Check sheet for the modelled part. Datum: model origin and axes. Units: mm. A direction names the side the tool comes from. Give positions to 0.01 mm unless a question says otherwise; leave off trailing zeros. Order: outer loops, then holes, each group sorted by start corner. A loop starts at its lowest first (then second) coordinate and runs counter-clockwise, first axis right, second up. Notation, with made-up numbers: M -33,18 L 4,18 A11 ccw 4,29 Z; hole C 58,48 d8. An arc over 180 degrees is marked long. Return JSON: item names as keys, results as strings. Group by question number.
from build123d import *

# Parameters (mm, degrees)
SKETCH1_W           = 6.35
SKETCH1_H           = 19.05
BOSS_EXTRUDE1_DEPTH = 1.5875
SKETCH2_W           = 5.2832
SKETCH2_H           = 4.7625
CUT_EXTRUDE1_DEPTH  = 1.5875
SKETCH3_R           = 0.762
SKETCH3_R_2         = 1.2573
CUT_EXTRUDE2_DEPTH  = 3.175
SKETCH31_R          = 2.54
CUT_EXTRUDE5_DEPTH  = 1.778


with BuildPart() as part:
    # Sketch1 → Boss-Extrude1 (new body, symmetric)
    with BuildSketch(Plane(origin=(0, 0, 0), x_dir=(1, 0, 0), z_dir=(0, 1, 0))):
        Polygon((-3.175, 15.08125), (-14.44625, 15.08125), (-14.44625, -15.08125), (-9.16305, -15.08125), (-9.16305, 5.55625), (9.16305, 5.55625), (9.16305, -15.08125), (14.44625, -15.08125), (14.44625, 15.08125), (3.175, 15.08125), align=None)
        with Locations((0, 24.60625)):
            Rectangle(SKETCH1_W, SKETCH1_H)
    extrude(amount=BOSS_EXTRUDE1_DEPTH, both=True)

    # Sketch2 → Cut-Extrude1 (cut)
    with BuildSketch(Plane(origin=(0, 1.5875, 0), x_dir=(1, 0, 0), z_dir=(0, 1, 0))):
        with Locations((-11.80465, -12.7)):
            Rectangle(SKETCH2_W, SKETCH2_H)
        with Locations((11.80465, -12.7)):
            Rectangle(SKETCH2_W, SKETCH2_H)
    extrude(amount=-CUT_EXTRUDE1_DEPTH, mode=Mode.SUBTRACT)

    # Sketch3 → Cut-Extrude2 (cut)
    with BuildSketch(Plane(origin=(0, 1.5875, 0), x_dir=(1, 0, 0), z_dir=(0, 1, 0))):
        with Locations((-11.65225, -12.7)):
            Circle(SKETCH3_R)
        with Locations((11.65225, -12.7)):
            Circle(SKETCH3_R)
        with Locations((0, 17.294029814)):
            Circle(SKETCH3_R_2)
        with Locations((0, 29.994029814)):
            Circle(SKETCH3_R_2)
    extrude(amount=-CUT_EXTRUDE2_DEPTH, mode=Mode.SUBTRACT)

    # Sketch31 → Cut-Extrude5 (cut)
    with BuildSketch(Plane(origin=(0, 1.5875, 0), x_dir=(1, 0, 0), z_dir=(0, 1, 0))):
        with Locations((0, 17.294029814)):
            Circle(SKETCH31_R)
        with Locations((0, 29.994029814)):
            Circle(SKETCH31_R)
    extrude(amount=-CUT_EXTRUDE5_DEPTH, mode=Mode.SUBTRACT)


solid = part.part
1) Sectioned sample at A-A on z = 12.7. Record the boundary of the cut face in (x, y), then the cut area to 3 significant figures.
2) Sectioned sample at C-C on y = 0.6. Record the boundary of the cut face in (x, z) (3 decimals), then the cut area to 3 significant figures.
3) Material ranges on line 1 along Z through (x, y) = (0, 1.15); line 2 along X through (y, z) = (-0.6, 12.7); line 3 along X through (y, z) = (1, -5.5), recorded low to high.
4) Sectioned sample at B-B on x = 0. Record the boundary of the cut face in (y, z).
5) Depth check by flat-ended pin: P1, Ø2.5, axis at x = -11.5, z = 13, coming from the +Y side; P2, Ø1.7, axis at x = 12, y = 1, coming from the +Z side; P3, Ø3, axis at x = 0, z = -17.29, coming from the +Y side. Enter the tip coordinate at first touch or a pass-through.
6) Tool access check on faces 1 (the face through (-0.331, 0.711, -32.512)), 2 (the face through (-3.175, 0, -24)), 3 (the face through (12, 1, 10.319)), 4 (the face through (3.175, 0, -24)), 5 (the face through (0, 0, -5.556)). Record the directions out of +Z, -Z, +X, -X, +Y, -Y that give a thin tool (end or side, any length) a straight path to the whole face; none if there is none.
7) Sectioned sample at D-D on x = 9.75. Record the boundary of the cut face in (y, z).
8) Release check for a two-part mould opening along X. For faces 6 (the face through (-14.446, 0, 0)), 7 (the face through (-1, -0.191, -29)), 8 (the face through (-12, 1, 10.319)), 9 (the face through (14.446, 0, 0)) record: released by +X, released by -X, zero draft, split by the parting line, or undercut.
Reply:
{
 "1": {"outline": "M -14.45,-1.59 L -12.41,-1.59 L -12.41,0 L -14.45,0 Z; M -10.89,-1.59 L -9.16,-1.59 L -9.16,0 L -10.89,0 Z; M 9.16,-1.59 L 10.89,-1.59 L 10.89,0 L 9.16,0 Z; M 12.41,-1.59 L 14.45,-1.59 L 14.45,0 L 12.41,0 Z", "area": "11.9 mm^2"},
 "2": {"outline": "M -14.446,-15.081 L -3.175,-15.081 L -3.175,-34.131 L 3.175,-34.131 L 3.175,-15.081 L 14.446,-15.081 L 14.446,10.319 L 9.163,10.319 L 9.163,-5.556 L -9.163,-5.556 L -9.163,10.319 L -14.446,10.319 Z; hole C 0,-29.994 d5.08; hole C 0,-17.294 d5.08", "area": "523 mm^2"},
 "3": {"line 1": "-34.13 to -32.53, -27.45 to -19.83, -14.75 to -5.56", "line 2": "-14.45 to -12.41, -10.89 to -9.16, 9.16 to 10.89, 12.41 to 14.45", "line 3": "-14.45 to -9.16, 9.16 to 14.45"},
 "4": {"outline": "M -1.59,-34.13 L 1.59,-34.13 L 1.59,-32.53 L -0.19,-32.53 L -0.19,-31.25 L -1.59,-31.25 Z; M -1.59,-28.74 L -0.19,-28.74 L -0.19,-27.45 L 1.59,-27.45 L 1.59,-19.83 L -0.19,-19.83 L -0.19,-18.55 L -1.59,-18.55 Z; M -1.59,-16.04 L -0.19,-16.04 L -0.19,-14.75 L 1.59,-14.75 L 1.59,-5.56 L -1.59,-5.56 Z"},
 "5": {"P1": "y = 0", "P2": "z = 10.32", "P3": "y = -0.19"},
 "6": {"face 1": "+Y", "face 2": "-Z, -X, +Y, -Y", "face 3": "+Z, +X, -X, +Y", "face 4": "-Z, +X, +Y, -Y", "face 5": "+Z, +Y, -Y"},
 "7": {"outline": "M -1.59,-15.08 L 1.59,-15.08 L 1.59,10.32 L 0,10.32 L 0,15.08 L -1.59,15.08 Z"},
 "8": {"face 6": "released by -X", "face 7": "undercut", "face 8": "zero draft", "face 9": "released by +X"}
}
